```python
from build123d import *

# Parameters (mm, degrees)
SKETCH1_R           = 8.8
SKETCH1_R_2         = 6.3
BOSS_EXTRUDE1_DEPTH = 4
CHAMFER1_SIZE       = 0.5
CHAMFER2_SIZE       = 0.5


with BuildPart() as part:
    # Sketch1 → Boss-Extrude1 (new body)
    with BuildSketch(Plane(origin=(0, 0, 0), x_dir=(0, 0, -1), z_dir=(1, 0, 0))):
        Circle(SKETCH1_R)
        Circle(SKETCH1_R_2, mode=Mode.SUBTRACT)
    extrude(amount=BOSS_EXTRUDE1_DEPTH)

    # Chamfer1
    chamfer1_edges = [part.edges().sort_by_distance(p)[0] for p in [
        (0, 0, 8.8),
        (4, 0, 8.8),
    ]]
    chamfer(chamfer1_edges, length=CHAMFER1_SIZE)

    # Chamfer2
    chamfer2_edges = [part.edges().sort_by_distance(p)[0] for p in [
        (0, 0, 6.3),
        (4, 0, 6.3),
    ]]
    chamfer(chamfer2_edges, length=CHAMFER2_SIZE)


solid = part.part
```
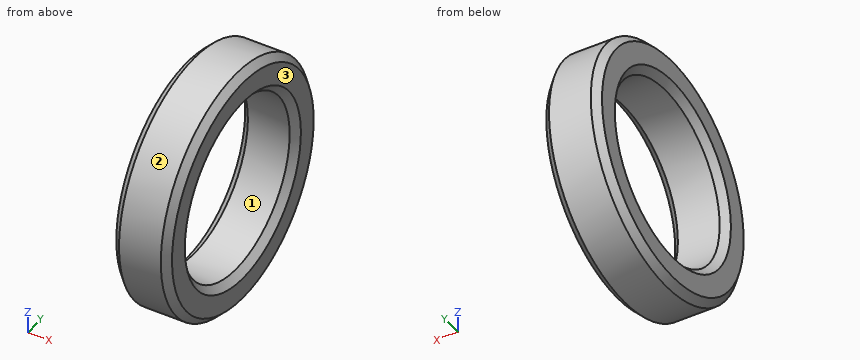
Check sheet for the modelled part. Datum: model origin and axes. Units: mm. Face numbers are marked on the shaded views. Round coordinates to 2 decimals unless told otherwise and drop trailing zeros. Loops run counter-clockwise (first coordinate to the right, second up) from the corner with the lowest first, then second, coordinate; pieces in that order, holes last. Notation, with made-up numbers: M 18,-13.75 L 25,-13.75 A28 cw 25,6.25 Z; hole C -23,9 d2. An arc over 180 degrees is marked long. Answer as a JSON object with one key per item and string values.
1. Scan lines: line 1 (Y direction, x = 2.75, z = -0.25); line 2 (Y direction, x = 1.25, z = -4.5); line 3 (Z direction, x = 2.1, y = 1.75). Record each from-to range of solid material in increasing order.
Reply:
{"line 1": "y = -8.8 to -6.3, 6.3 to 8.8", "line 2": "y = -7.56 to -4.41, 4.41 to 7.56", "line 3": "z = -8.62 to -6.05, 6.05 to 8.62"}
2. Mould release check, pull along Y, two halves, no side actions. Record for the marked faces 1, 2 and 3: pulls with the +Y half, pulls with the -Y half, needs draft (parallel to the pull), parting line crosses it, or undercut.
Reply:
{"face 1": "undercut", "face 2": "parting line crosses it", "face 3": "needs draft"}
3. Section check A-A (z = 0). Record the boundary of the cut face in (x, y).
Reply:
{"outline": "M 0,-8.3 L 0.5,-8.8 L 3.5,-8.8 L 4,-8.3 L 4,-6.8 L 3.5,-6.3 L 0.5,-6.3 L 0,-6.8 Z; M 0,6.8 L 0.5,6.3 L 3.5,6.3 L 4,6.8 L 4,8.3 L 3.5,8.8 L 0.5,8.8 L 0,8.3 Z"}
4. Gauge pin test, flat end, axial feed: P1, Ø1, axis at x = 2.5, z = 6, coming from the +Y side. Record the tip position at first contact, or that the pin passes through.
Reply:
{"P1": "stops at y = 6.87"}
5. Section check C-C (x = 2.05). Record the boundary of the cut face in (y, z), plus the area to 3 significant figures.
Reply:
{"outline": "C 0,0 d17.6; hole C 0,0 d12.6", "area": "119 mm²"}
